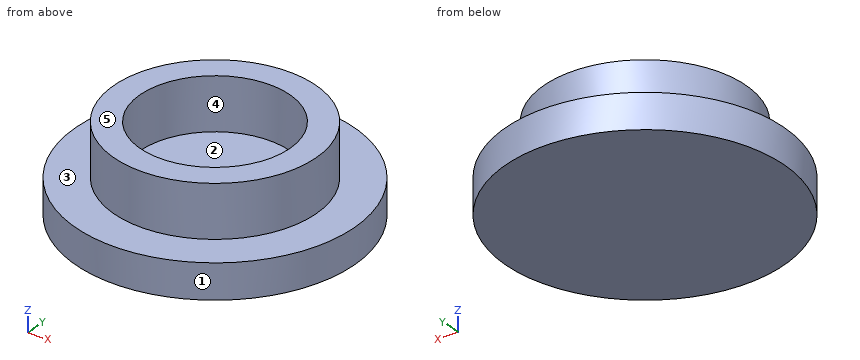
from build123d import *

# Parameters (mm, degrees)
F0_R     = 5.8
F0_R_2   = 4.3
F1_DEPTH = 3
F0_R_3   = 8
F2_DEPTH = 2


with BuildPart() as f1:
    # F0 (on Top) → F1 (new body)
    with BuildSketch(Plane.XY):
        Circle(F0_R)
        Circle(F0_R_2, mode=Mode.SUBTRACT)
    extrude(amount=F1_DEPTH)

    # F0 (on Top) → F2 (join)
    with BuildSketch(Plane.XY):
        Circle(F0_R_3)
        Circle(F0_R, mode=Mode.SUBTRACT)
        Circle(F0_R)
        Circle(F0_R_2, mode=Mode.SUBTRACT)
        Circle(F0_R_2)
    extrude(amount=-F2_DEPTH)


solid = f1.part
Verification items for the finished model (mm, model axes). Face numbers are marked on the shaded views. A direction names the side the tool comes from. Coordinates: 2 decimals unless noted, no trailing zeros. Order: outer loops, then holes, each group sorted by start corner. A loop starts at its lowest first (then second) coordinate and runs counter-clockwise, first axis right, second up.
Item 1: Depth check by flat-ended pin: pin 1 (1.5 mm diameter, centred on x = 4, y = 1.5, fed in from +Z). Enter the tip coordinate at first touch or a pass-through.
Filled in:
pin 1: stops at z = 3
Item 2: Section check A-A, the plane x = 0. Enter the section's corners in (y, z), then the cut area to 3 significant figures.
Filled in:
outline: (-8, -2) - (8, -2) - (8, 0) - (5.8, 0) - (5.8, 3) - (4.3, 3) - (4.3, 0) - (-4.3, 0) - (-4.3, 3) - (-5.8, 3) - (-5.8, 0) - (-8, 0) - close
area: 41.0 mm2
Item 3: Access from +Z, -Z, +X, -X, +Y, -Y to the whole of each face (thin tool, end or side, straight path). Record for the marked faces 4 and 5.
Filled in:
face 4: +Z
face 5: +Z, +X, -X, +Y, -Y
Item 4: Section check D-D, the plane z = -1.25. Enter the section's corners in (x, y), then the cut area to 3 significant figures.
Filled in:
outline: circle Ø16 at (0, 0)
area: 201 mm2
Item 5: Material ranges on L1, parallel to Y at x = 0, z = 1.3; L2, parallel to Z at x = 3.75, y = -6.5; L3, parallel to Y at x = -3.25, z = 1.75, recorded low to high.
Filled in:
L1: y = -5.8 to -4.3, 4.3 to 5.8
L2: z = -2 to 0
L3: y = -4.8 to -2.82, 2.82 to 4.8
Item 6: Section check C-C, the plane z = 1.4. Enter the section's corners in (x, y).
Filled in:
outline: circle Ø11.6 at (0, 0); hole circle Ø8.6 at (0, 0)
Item 7: Release check for a two-part mould opening along Y. For the marked faces 1, 2 and 3 record: +Y half, -Y half, draft (parallel to the pull), parting line (faces both ways), or undercut.
Filled in:
face 1: parting line
face 2: undercut
face 3: draft
